Part model, mm, in its own coordinate system. Coordinates: 2 decimals unless noted, no trailing zeros. Order: outer loops, then holes, each group sorted by start corner. A loop starts at its lowest first (then second) coordinate and runs counter-clockwise, first axis right, second up.
from build123d import *

# Parameters (mm, degrees)
F1_DEPTH = 63.5
F2_R     = 25.4


with BuildPart() as f1:
    # F0 (on Right) → F1 (new body, symmetric)
    with BuildSketch(Plane.YZ):
        Polygon((-61.47124, -33.72718), (-1.527025, -70.099246), (59.944215, -36.372065), (61.47124, 33.72718), (1.527025, 70.099246), (-59.944215, 36.372065), align=None)
    extrude(amount=F1_DEPTH, both=True)

    # F2
    f2_edges = [f1.edges().sort_by_distance(p)[0] for p in [
        (0, -59.944215, 36.372065),
    ]]
    fillet(f2_edges, radius=F2_R)


solid = f1.part
Q1. Wall check: line 1 along Z through (x, y) = (24, 31); line 2 along Z through (x, y) = (0, 27); line 3 along Y through (x, z) = (33, -55). Give the ranges that are in metal, low to high.
Results list:
line 1: z = -52.25 to 52.22
line 2: z = -54.45 to 54.64
line 3: y = -26.41 to 25.99
Q2. Pin check, flat tips, straight feed: pin 1 Ø6 at (x, y) = (-9.5, 27) entering from -Z; pin 2 Ø12 at (x, z) = (-35, -51.5) entering from -Y; pin 3 Ø12 at (x, y) = (1, -17.5) entering from -Z. Stop position of each tip, or through.
Results list:
pin 1: stops at z = -56.09
pin 2: stops at y = -42.07
pin 3: stops at z = -64.05
Q3. Mould opens along Y. For faces 1 (the face through (-0.889, -56.681, 34.174)), 2 (the face through (0.89, 31.92, 51.66)), 3 (the face through (-63.5, -1, 1)) say: pulls with the +Y half, pulls with the -Y half, needs draft (parallel to the pull), parting line crosses it, or undercut.
Results list:
face 1: pulls with the -Y half
face 2: pulls with the +Y half
face 3: needs draft
Q4. Cut at A-A on x = -1. Write the cut outline in (y, z), and give its area (3 significant figures).
Results list:
outline: (-61.47, -33.73) - (-1.53, -70.1) - (59.94, -36.37) - (61.47, 33.73) - (1.53, 70.1) - (-47.09, 43.43) arc R25.4 ccw to (-60.26, 21.71) - close
area: 12,700 mm2
Q5. Cut at C-C on z = 60. Write the cut outline in (x, y).
Results list:
outline: (-63.5, -16.88) - (63.5, -16.88) - (63.5, 18.17) - (-63.5, 18.17) - close
Q6. Cut at B-B on y = 5.5. Write the cut outline in (x, z).
Results list:
outline: (-63.5, -66.24) - (63.5, -66.24) - (63.5, 67.69) - (-63.5, 67.69) - close
